Geometry check sheet. Reference: the model listing, model coordinates, mm. A direction names the side the tool comes from. Give positions to 0.01 mm unless a question says otherwise; leave off trailing zeros. Loops run counter-clockwise (first coordinate to the right, second up) from the corner with the lowest first, then second, coordinate; pieces in that order, holes last. Notation, with made-up numbers: (34, -12.75) -> (51, -12.75) arc R27 ccw to (51, 15.25) -> close; hole circle Ø10 at (44.25, -1.75). An arc over 180 degrees is marked (long way). One line per question, with ' | ' between items.
from build123d import *

# Parameters (mm, degrees)
ESBO_O4_R                = 4.3
RESSALTO_EXTRUS_O1_DEPTH = 25
ESBO_O5_W                = 7
ESBO_O5_H                = 4
RESSALTO_EXTRUS_O4_DEPTH = 3
ESBO_O7_W                = 2.98
ESBO_O7_H                = 4
CORTE_EXTRUS_O2_DEPTH    = 3
ESBO_O8_R                = 0.9
CORTE_EXTRUS_O3_DEPTH    = 2
FILETE2_RADIUS           = 2
FILETE2_LENGTH           = 2.01
FILETE3_RADIUS           = 2
FILETE3_LENGTH           = 2.01
FILETE4_R                = 0.5


with BuildPart() as part:
    # Esboço4 → Ressalto-extrusão1 (new body)
    with BuildSketch(Plane(origin=(0, 0, 0), x_dir=(0, 0, -1), z_dir=(1, 0, 0))):
        Circle(ESBO_O4_R)
    extrude(amount=-RESSALTO_EXTRUS_O1_DEPTH)

    # Esboço5 → Ressalto-extrusão4 (add)
    with BuildSketch(Plane.ZY.offset(25)):
        Rectangle(ESBO_O5_W, ESBO_O5_H)
    extrude(amount=RESSALTO_EXTRUS_O4_DEPTH)

    # Esboço7 → Corte-extrusão2 (cut)
    with BuildSketch(Plane.ZY.offset(28)):
        Rectangle(ESBO_O7_W, ESBO_O7_H)
    extrude(amount=-CORTE_EXTRUS_O2_DEPTH, mode=Mode.SUBTRACT)

    # Esboço8 → Corte-extrusão3 (cut)
    with BuildSketch(Plane.XY.offset(-1.49)):
        with Locations((-26.63, 0)):
            Circle(ESBO_O8_R)
    corte_extrus_o3 = extrude(amount=-CORTE_EXTRUS_O3_DEPTH, mode=Mode.SUBTRACT)

    # Filete2: full round fillet: the end face becomes a half cylinder, R = half its width
    filete2_face = Plane((-28, 0, -2.495), x_dir=(0, 0, -1), z_dir=(-1, 0, 0))  # on the end face: x along it, z out of the body
    filete2_slab = filete2_face.offset(-FILETE2_RADIUS / 2) * Box(FILETE2_LENGTH, 2 * FILETE2_RADIUS, FILETE2_RADIUS, mode=Mode.PRIVATE)  # the body's end, R deep
    filete2_round = Plane((-26, 0, -2.495), x_dir=(-1, 0, 0), z_dir=(0, 0, -1)) * Cylinder(FILETE2_RADIUS, FILETE2_LENGTH, mode=Mode.PRIVATE)  # its axis R under the face
    add(filete2_slab - filete2_round, mode=Mode.SUBTRACT)

    # Espelhar7: Corte-extrusão3 across plane
    add(corte_extrus_o3.mirror(Plane.XY), mode=Mode.SUBTRACT)

    # Filete3: full round fillet: the end face becomes a half cylinder, R = half its width
    filete3_face = Plane((-28, 0, 2.495), x_dir=(0, 0, 1), z_dir=(-1, 0, 0))  # on the end face: x along it, z out of the body
    filete3_slab = filete3_face.offset(-FILETE3_RADIUS / 2) * Box(FILETE3_LENGTH, 2 * FILETE3_RADIUS, FILETE3_RADIUS, mode=Mode.PRIVATE)  # the body's end, R deep
    filete3_round = Plane((-26, 0, 2.495), x_dir=(-1, 0, 0), z_dir=(0, 0, 1)) * Cylinder(FILETE3_RADIUS, FILETE3_LENGTH, mode=Mode.PRIVATE)  # its axis R under the face
    add(filete3_slab - filete3_round, mode=Mode.SUBTRACT)

    # Filete4
    # the kernel refuses this fillet: 0.5 mm, written as the material it takes off along each edge
    with BuildSketch(Plane(origin=(-25, 0, 0), x_dir=(0, 0, -1), z_dir=(0, -1, 0))) as filete4_piece_1_section:
        with BuildLine():
            CenterArc((4.3 - FILETE4_R, FILETE4_R), FILETE4_R, 270, 90)
            Line((4.3 - FILETE4_R, 0), (4.3, 0))
            Line((4.3, 0), (4.3, FILETE4_R))
        make_face()
    filete4_piece_1 = revolve(axis=Axis((-25, 0, 0), (1, 0, 0)), mode=Mode.PRIVATE)
    filete4_piece_1 = split(filete4_piece_1, bisect_by=Plane(origin=(-24.857838708, 1.067183876, -3.5), z_dir=(0, 0, -1)), keep=Keep.TOP, mode=Mode.PRIVATE)
    add(filete4_piece_1, mode=Mode.SUBTRACT)
    with BuildSketch(Plane(origin=(-25, 0, 0), x_dir=(0, 0, -1), z_dir=(0, -1, 0))) as filete4_piece_2_section:
        with BuildLine():
            CenterArc((4.3 - FILETE4_R, FILETE4_R), FILETE4_R, 270, 90)
            Line((4.3 - FILETE4_R, 0), (4.3, 0))
            Line((4.3, 0), (4.3, FILETE4_R))
        make_face()
    filete4_piece_2 = revolve(axis=Axis((-25, 0, 0), (1, 0, 0)), mode=Mode.PRIVATE)
    filete4_piece_2 = split(filete4_piece_2, bisect_by=Plane(origin=(-24.858947412, 2, 0), z_dir=(0, 1, 0)), keep=Keep.TOP, mode=Mode.PRIVATE)
    add(filete4_piece_2, mode=Mode.SUBTRACT)
    with BuildSketch(Plane(origin=(-25, 0, 0), x_dir=(0, 0, -1), z_dir=(0, -1, 0))) as filete4_piece_3_section:
        with BuildLine():
            CenterArc((4.3 - FILETE4_R, FILETE4_R), FILETE4_R, 270, 90)
            Line((4.3 - FILETE4_R, 0), (4.3, 0))
            Line((4.3, 0), (4.3, FILETE4_R))
        make_face()
    filete4_piece_3 = revolve(axis=Axis((-25, 0, 0), (1, 0, 0)), mode=Mode.PRIVATE)
    filete4_piece_3 = split(filete4_piece_3, bisect_by=Plane(origin=(-24.858947412, -2, 0), z_dir=(0, -1, 0)), keep=Keep.TOP, mode=Mode.PRIVATE)
    add(filete4_piece_3, mode=Mode.SUBTRACT)
    with BuildSketch(Plane(origin=(-25, 0, 0), x_dir=(0, 0, -1), z_dir=(0, -1, 0))) as filete4_piece_4_section:
        with BuildLine():
            CenterArc((4.3 - FILETE4_R, FILETE4_R), FILETE4_R, 270, 90)
            Line((4.3 - FILETE4_R, 0), (4.3, 0))
            Line((4.3, 0), (4.3, FILETE4_R))
        make_face()
    filete4_piece_4 = revolve(axis=Axis((-25, 0, 0), (1, 0, 0)), mode=Mode.PRIVATE)
    filete4_piece_4 = split(filete4_piece_4, bisect_by=Plane(origin=(-24.85783871, 0, 3.5), z_dir=(0, 0, 1)), keep=Keep.TOP, mode=Mode.PRIVATE)
    add(filete4_piece_4, mode=Mode.SUBTRACT)


solid = part.part
Item 1: Scan lines: probe 1 along Y at (x, z) = (-13.75, 2.5); probe 2 along Y at (x, z) = (-26.63, 2.2); probe 3 along Y at (x, z) = (-19, 3.5). Record each from-to range of solid material in increasing order.
Result:
probe 1: -3.5 to 3.5 | probe 2: -1.9 to -0.9, 0.9 to 1.9 | probe 3: -2.5 to 2.5
Item 2: Depth check by flat-ended pin: pin 1 Ø0.9 at (x, y) = (-26, -1) entering from +Z; pin 2 Ø0.9 at (x, y) = (-27, 0) entering from -Z; pin 3 Ø0.5 at (x, z) = (-25.5, 2) entering from -Y; pin 4 Ø4 at (y, z) = (2.5, -3.5) entering from +X. Enter the tip coordinate at first touch or a pass-through.
Result:
pin 1: z = 3.5 | pin 2: z = -3.5 | pin 3: y = -2 | pin 4: x = 0
Item 3: Sectioned sample at D-D (x = -2.25). Record the cut outline in (y, z).
Result:
outline: circle Ø8.6 at (0, 0)
Item 4: Release check for a two-part mould opening along X. For faces 4 (the face through (-27.53, 0.04, 2.48)), 5 (the face through (-28, 0, 3)), 6 (the face through (0, 0, 0)), 7 (the face through (-25.5, 0, -1.49)) record: pulls with the +X half, pulls with the -X half, needs draft (parallel to the pull), parting line crosses it, or undercut.
Result:
face 4: undercut | face 5: pulls with the -X half | face 6: pulls with the +X half | face 7: needs draft
Item 5: Set-up check for faces 1 (the face through (-12.078, 0.189, 4.296)), 2 (the face through (-27.53, 0.04, -2.48)), 3 (the face through (-25.5, 0, 1.49)): record each of +Z, -Z, +X, -X, +Y, -Y from which the full face is reachable in a straight line by a thin tool's end or side.
Result:
face 1: +X, -X | face 2: none | face 3: -X, +Y, -Y
Item 6: Sectioned sample at A-A (x = -26.63). Record the cut outline in (y, z), plus the area to 3 significant figures.
Result:
outline: (-1.9, -3.5) -> (1.9, -3.5) -> (1.9, -1.49) -> (0.9, -1.49) -> (0.9, -3.49) -> (-0.9, -3.49) -> (-0.9, -1.49) -> (-1.9, -1.49) -> close; (-1.9, 1.49) -> (-0.9, 1.49) -> (-0.9, 3.49) -> (0.9, 3.49) -> (0.9, 1.49) -> (1.9, 1.49) -> (1.9, 3.5) -> (-1.9, 3.5) -> close | area: 8.06 mm2
Item 7: Sectioned sample at C-C (z = 0). Record the cut outline in (x, y), plus the area to 3 significant figures.
Result:
outline: (-25, -3.8) arc R0.5 ccw to (-24.5, -4.3) -> (0, -4.3) -> (0, 4.3) -> (-24.5, 4.3) arc R0.5 ccw to (-25, 3.8) -> close | area: 215 mm2
Item 8: Sectioned sample at B-B (y = 0). Record the cut outline in (x, z), plus the area to 3 significant figures.
Result:
outline: (-28, -3.5) -> (-25, -3.5) -> (-25, -3.8) arc R0.5 ccw to (-24.5, -4.3) -> (0, -4.3) -> (0, 4.3) -> (-24.5, 4.3) arc R0.5 ccw to (-25, 3.8) -> (-25, 3.5) -> (-28, 3.5) -> (-28, 1.49) -> (-27.53, 1.49) -> (-27.53, 3.49) -> (-25.73, 3.49) -> (-25.73, 1.49) -> (-25, 1.49) -> (-25, -1.49) -> (-25.73, -1.49) -> (-25.73, -3.49) -> (-27.53, -3.49) -> (-27.53, -1.49) -> (-28, -1.49) -> close | area: 220 mm2
